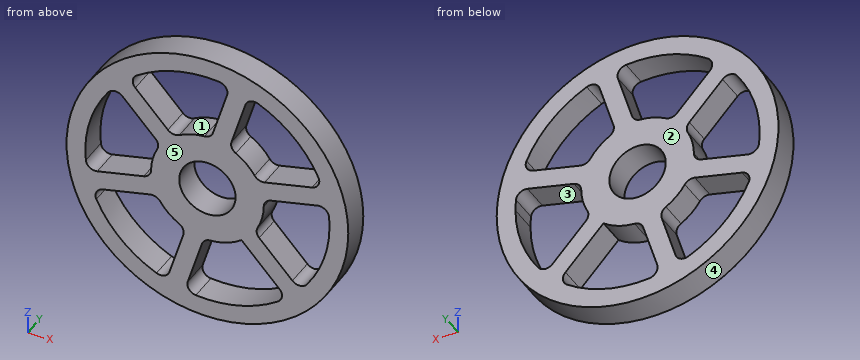
```python
from build123d import *

# Parameters (mm, degrees)
F0_R     = 75
F0_R_2   = 15
F1_DEPTH = 15
F3_DEPTH = 25
F4_R     = 5
F5_R     = 5


with BuildPart() as f1:
    # F0 (on Front) → F1 (new body)
    with BuildSketch(Plane.XZ):
        Circle(F0_R)
        Circle(F0_R_2, mode=Mode.SUBTRACT)
    extrude(amount=-F1_DEPTH)

    # F2 (on face) → F3 (cut)
    with BuildSketch(Plane.XZ):
        with BuildLine():
            ThreePointArc((-29.761636, -3.774261), (-29.2124, 6.829033), (-25.004101, 16.57694))
            Line((-25.004101, 16.57694), (-49.222236, 42.45199))
            ThreePointArc((-49.222236, 42.45199), (-62.729048, 17.031339), (-63.932898, -11.729645))
            Line((-63.932898, -11.729645), (-29.761636, -3.774261))
        make_face()
        with BuildLine():
            ThreePointArc((-18.149424, 23.887202), (-8.692084, 28.713197), (1.854001, 29.942657))
            Line((1.854001, 29.942657), (12.153383, 63.853702))
            ThreePointArc((12.153383, 63.853702), (-16.614952, 62.840619), (-42.12462, 49.502691))
            Line((-42.12462, 49.502691), (-18.149424, 23.887202))
        make_face()
        with BuildLine():
            ThreePointArc((11.612212, 27.661463), (20.520316, 21.884164), (26.858102, 13.365716))
            Line((26.858102, 13.365716), (61.37562, 21.401712))
            ThreePointArc((61.37562, 21.401712), (46.114096, 45.80928), (21.808278, 61.232336))
            Line((21.808278, 61.232336), (11.612212, 27.661463))
        make_face()
        with BuildLine():
            ThreePointArc((29.761636, 3.774261), (29.94035, 1.89089), (30, 0))
            ThreePointArc((30, 0), (28.723884, -8.656702), (25.004101, -16.57694))
            Line((25.004101, -16.57694), (49.222236, -42.45199))
            ThreePointArc((49.222236, -42.45199), (60.928012, -22.644587), (65, 0))
            ThreePointArc((65, 0), (64.732675, 5.889043), (63.932898, 11.729645))
            Line((63.932898, 11.729645), (29.761636, 3.774261))
        make_face()
        with BuildLine():
            Line((42.12462, -49.502691), (18.149424, -23.887202))
            ThreePointArc((18.149424, -23.887202), (8.692084, -28.713197), (-1.854001, -29.942657))
            Line((-1.854001, -29.942657), (-12.153383, -63.853702))
            ThreePointArc((-12.153383, -63.853702), (16.614952, -62.840619), (42.12462, -49.502691))
        make_face()
        with BuildLine():
            Line((-21.808278, -61.232336), (-11.612212, -27.661463))
            ThreePointArc((-11.612212, -27.661463), (-20.520316, -21.884164), (-26.858102, -13.365716))
            Line((-26.858102, -13.365716), (-61.37562, -21.401712))
            ThreePointArc((-61.37562, -21.401712), (-46.114096, -45.80928), (-21.808278, -61.232336))
        make_face()
    extrude(amount=-F3_DEPTH, mode=Mode.SUBTRACT)

    # F4
    f4_edges = [f1.edges().sort_by_distance(p)[0] for p in [
        (-63.932898, 7.5, -11.729645),
        (-49.222236, 7.5, 42.45199),
        (12.153383, 7.5, 63.853702),
        (-42.12462, 7.5, 49.502691),
        (21.808278, 7.5, 61.232336),
        (61.37562, 7.5, 21.401712),
        (63.932898, 7.5, 11.729645),
        (49.222236, 7.5, -42.45199),
        (42.12462, 7.5, -49.502691),
        (-12.153383, 7.5, -63.853702),
        (-21.808278, 7.5, -61.232336),
        (-61.37562, 7.5, -21.401712),
    ]]
    fillet(f4_edges, radius=F4_R)

    # F5
    f5_edges = [f1.edges().sort_by_distance(p)[0] for p in [
        (25.004101, 7.5, -16.57694),
        (29.761636, 7.5, 3.774261),
        (-1.854001, 7.5, -29.942657),
        (-11.612212, 7.5, -27.661463),
        (-26.858102, 7.5, -13.365716),
        (-29.761636, 7.5, -3.774261),
        (-25.004101, 7.5, 16.57694),
        (-18.149424, 7.5, 23.887202),
        (1.854001, 7.5, 29.942657),
        (11.612212, 7.5, 27.661463),
        (26.858102, 7.5, 13.365716),
    ]]
    fillet(f5_edges, radius=F5_R)


solid = f1.part
```
Build history of the part. All positions in model axes, mm. Face numbers are marked on the shaded views. A direction names the side the tool comes from. Give positions to 0.01 mm unless a question says otherwise; leave off trailing zeros. Loops run counter-clockwise (first coordinate to the right, second up) from the corner with the lowest first, then second, coordinate; pieces in that order, holes last.
Item 1: Drill centre lines: line 1 (X direction, y = 5, z = 50.5); line 2 (Z direction, x = 43, y = 14.5); line 3 (X direction, y = 4.5, z = 20.5). Where is each one in solid material? Low to high.
Answers follow:
line 1: x = -55.45 to -39.48, 8.1 to 18.55, 40.92 to 55.45
line 2: z = -61.45 to -35.8, 6.86 to 17.12, 48.74 to 61.45
line 3: x = -72.14 to -61.68, -28.68 to 21.9, 56.85 to 72.14
Item 2: Slice it at D-D, the plane x = 22. List the corners of the cut face in (y, z), and give its area (3 significant figures).
Answers follow:
outline: (0, -71.7) - (15, -71.7) - (15, -61.16) - (0, -61.16) - close; (0, -28) - (15, -28) - (15, 20.4) - (0, 20.4) - close; (0, 58.54) - (15, 58.54) - (15, 71.7) - (0, 71.7) - close
area: 1,080 mm2
Item 3: Slice it at C-C, the plane y = 7. Give the number of separate pieces and of enclosed holes in the cut face, and give its area (3 significant figures).
Answers follow:
separate pieces: 1
enclosed holes: 7
area: 8,750 mm2
Item 4: Flat gauge pins, fed straight in: pin 1 (3 mm diameter, centred on y = 2.5, z = 25.5, fed in from -X); pin 2 (5 mm diameter, centred on y = 9.5, z = 35.5, fed in from -X); pin 3 (8 mm diameter, centred on y = 3, z = 24.5, fed in from -X). Where does each tip first touch, or does it go through?
Answers follow:
pin 1: stops at x = -71.06
pin 2: stops at x = -67.35
pin 3: stops at x = -72.14
Item 5: Slice it at A-A, the plane z = -43. List the corners of the cut face in (x, y), and give its area (3 significant figures).
Answers follow:
outline: (-61.45, 0) - (-48.74, 0) - (-48.74, 15) - (-61.45, 15) - close; (-16.27, 0) - (-5.82, 0) - (-5.82, 15) - (-16.27, 15) - close; (36.04, 0) - (61.45, 0) - (61.45, 15) - (36.04, 15) - close
area: 729 mm2
Item 6: Which spindle directions (+Z, -Z, +X, -X, +Y, -Y) get a long thin tool onto all of the face, cutting with end or side? Do the marked faces 1 and 2. Say none if no direction does.
Answers follow:
face 1: +Y, -Y
face 2: +Z, -Z, +X, -X, +Y
Item 7: Pull direction X, two halves, no side cores. Call the marked faces 3, 4 and 5: released by +X, released by -X, zero draft, split by the parting line, or undercut.
Answers follow:
face 3: undercut
face 4: split by the parting line
face 5: zero draft
Item 8: Slice it at B-B, the plane x = 62. List the corners of the cut face in (y, z).
Answers follow:
outline: (0, -42.2) - (15, -42.2) - (15, -19.52) - (0, -19.52) - close; (0, 10.08) - (15, 10.08) - (15, 42.2) - (0, 42.2) - close
